Source: CAD feature listing. Evaluate the final solid. Frame: model axes, mm. A direction names the side the tool comes from. Round coordinates to 2 decimals unless told otherwise and drop trailing zeros. Write each loop counter-clockwise with the first axis right and the second up, starting at its lowest first coordinate (ties: lowest second). Pieces come first, ordered by that corner, then holes. Notation, with made-up numbers: (-3, 36) -> (47, 36) arc R21 ccw to (47, 44) -> close; hole circle Ø2 at (-37.5, 3). An arc over 180 degrees is marked (long way). Put each result on its own line as item: value.
Autodesk Inventor part; units mm, degrees
ref_plane "Work Plane1" through (0, 0, 0) normal (0, 0, 1) x (1, 0, 0)
ref_plane "YZ Plane" through (0, 0, 0) normal (1, 0, 0) x (0, 1, 0)
ref_plane "XZ Plane" through (0, 0, 0) normal (0, 1, 0) x (-1, 0, 0)
ref_plane "Work Plane1" through (0, 0, 0) normal (0, 0, 1) x (1, 0, 0)
sketch "Sketch1" plane through (0, 0, 0) normal (0, 0, 1) x (1, 0, 0)
  circle A0 centre (26.8, 19.857) radius 1.45
  circle A1 centre (26.8001, -10.143) radius 1.4501
  line L0 (26.8, 23.857) -> (24.8, 23.857)
  line L1 (24.8, 23.857) -> (23.8, 23.857)
  line L2 (23.8, 23.857) -> (23.8, -10.143)
  line L3 (23.8, -10.143) -> (23.8, -14.143)
  line L4 (23.8, -14.143) -> (26.8, -14.143)
  line L5 (26.8, -14.143) -> (29.8, -14.143)
  line L6 (29.8, -14.143) -> (29.8, 23.857)
  line L7 (29.8, 23.857) -> (26.8, 23.857)
  line L8 (26.8, 6.857) -> (29.8, 6.857)
  line L9 (26.8, 6.857) -> (23.8, 6.857)
  line L10 (26.8, -7.143) -> (23.8, -7.143)
  line L11 (26.8, -7.143) -> (29.8, -7.143)
  point P0 (0, 0)
  dimension "d0" = 4
  dimension "d1" = 2
  dimension "d2" = 1
  dimension "d3" = 4
  dimension "d4" = 3
  dimension "d6" = 3
extrude "Extrusion1" add sketch "Sketch1" along normal blind 1.5 contours L7 L6 L8 L9 L2 L1 L0 | L6 L5 L4 L3 L2 L10 L11
sketch "Sketch2" plane through (0, 0, 1.5) normal (0, 0, 1) x (1, 0, 0)
  line L0 (23.8, 23.857) -> (23.8, 6.857)
  line L1 (23.8, 6.857) -> (29.8, 6.857)
  line L2 (29.8, 6.857) -> (29.8, 23.857)
  line L3 (29.8, 23.857) -> (23.8, 23.857)
  circle A0 centre (26.8, 19.857) radius 1.45
  line L4 (23.8, 23.857) -> (23.8, -10.143)
  line L5 (29.8, -14.143) -> (29.8, 23.857)
  line L6 (29.8, -14.143) -> (29.8, -7.143)
  line L7 (29.8, -7.143) -> (23.8, -7.143)
  line L8 (23.8, -7.143) -> (23.8, -14.143)
  line L9 (23.8, -14.143) -> (29.8, -14.143)
  circle A1 centre (26.8001, -10.143) radius 1.4501
  point P0 (0, 0)
extrude "Extrusion2" add sketch "Sketch2" along normal blind 2
properties part number "gps_cable_holder"
Q1. Cut plane C-C on x = 29.45. Output: boundary loops of the cut face in (y, z).
Ans:
outline: (-14.14, 0) -> (-7.14, 0) -> (-7.14, 1.5) -> (6.86, 1.5) -> (6.86, 0) -> (23.86, 0) -> (23.86, 3.5) -> (-14.14, 3.5) -> close
Q2. Reachability of faces 4 (the flat face through (27, 15, 0)), 5 (the flat face through (27, -7.143, 1)) from +Z, -Z, +X, -X, +Y, -Y: full face, straight path, thin tool, end or side. Return the list, or none.
Ans:
face 4: -Z, +X, -X, +Y, -Y
face 5: -Z, +X, -X
Q3. Material intervals for line 1 (Y direction, x = 26.8, z = 1.1); line 2 (Y direction, x = 26.8, z = 2.65); line 3 (X direction, y = -10, z = 1.1), sorted ascending. Write a range as [from, to].
Ans:
line 1: y = [-14.14, -11.59], [-8.69, -7.14], [6.86, 18.41], [21.31, 23.86]
line 2: y = [-14.14, -11.59], [-8.69, 18.41], [21.31, 23.86]
line 3: x = [23.8, 25.36], [28.24, 29.8]
Q4. Draft query along X for faces 1 (the cylindrical face through (25.35, 19.79, 1.73)), 2 (the flat face through (27, 5, 3.5)), 3 (the flat face through (29.8, 5, 2)). Return one class per face: +X half, -X half, draft (parallel to the pull), parting line (faces both ways), or undercut.
Ans:
face 1: undercut
face 2: draft
face 3: +X half
Q5. Cut plane B-B on z = 0.75. Output: boundary loops of the cut face in (x, y).
Ans:
outline: (23.8, -14.14) -> (29.8, -14.14) -> (29.8, -7.14) -> (23.8, -7.14) -> close; (23.8, 6.86) -> (29.8, 6.86) -> (29.8, 23.86) -> (23.8, 23.86) -> close; hole circle Ø2.9 at (26.8, -10.14); hole circle Ø2.9 at (26.8, 19.86)
Q6. Cut plane A-A on x = 26.8. Output: boundary loops of the cut face in (y, z), and give its area (3 significant figures).
Ans:
outline: (-14.14, 0) -> (-11.59, 0) -> (-11.59, 3.5) -> (-14.14, 3.5) -> close; (-8.69, 0) -> (-7.14, 0) -> (-7.14, 1.5) -> (6.86, 1.5) -> (6.86, 0) -> (18.41, 0) -> (18.41, 3.5) -> (-8.69, 3.5) -> close; (21.31, 0) -> (23.86, 0) -> (23.86, 3.5) -> (21.31, 3.5) -> close
area: 91.7 mm^2
Q7. Cut plane D-D on z = 2.75. Output: boundary loops of the cut face in (x, y), and give its area (3 significant figures).
Ans:
outline: (23.8, -14.14) -> (29.8, -14.14) -> (29.8, 23.86) -> (23.8, 23.86) -> close; hole circle Ø2.9 at (26.8, -10.14); hole circle Ø2.9 at (26.8, 19.86)
area: 215 mm^2
Q8. Pin query (flat end, axial travel): pin 1 (1 mm diameter, centred on x = 28.5, y = 1.5, fed in from -Z). Return the tip coordinate at first contact, or that it passes through.
Ans:
pin 1: stops at z = 1.5
